Verification items for the finished model (mm, model axes). Round coordinates to 2 decimals unless told otherwise and drop trailing zeros. Order: outer loops, then holes, each group sorted by start corner. A loop starts at its lowest first (then second) coordinate and runs counter-clockwise, first axis right, second up. Notation, with made-up numbers: M 65.25,36.5 L 87.25,36.5 A18 cw 87.25,69.5 Z; hole C -28.5,-5.75 d7. An arc over 180 degrees is marked long. One line per item, written item: value. Start each with the question number.
from build123d import *

# Parameters (mm, degrees)
F1_DEPTH = 1.25
F2_R     = 2.5
F3_DEPTH = 2.501


# Not quite as in the source:
# - a feature names something its author has since deleted; it is built from what else it names


with BuildPart() as f1:
    # F0 (on Top) → F1 (new body, symmetric)
    with BuildSketch(Plane.XY):
        with BuildLine():
            Line((-5, 10), (-5, 0))
            Line((-5, 0), (5, 0))
            Line((5, 0), (5, 10))
            ThreePointArc((5, 10), (0, 5), (-5, 10))
        make_face()
        with BuildLine():
            Line((5, 0), (-5, 0))
            Line((-5, 0), (-5, -10))
            ThreePointArc((-5, -10), (0, -5), (5, -10))
            Line((5, -10), (5, 0))
        make_face()
        with BuildLine():
            ThreePointArc((5, 10), (0, 15), (-5, 10))
            ThreePointArc((-5, 10), (0, 5), (5, 10))
        make_face()
        with BuildLine():
            ThreePointArc((5, -10), (0, -5), (-5, -10))
            ThreePointArc((-5, -10), (0, -15), (5, -10))
        make_face()
    extrude(amount=F1_DEPTH, both=True)

    # F2 (on face) → F3 (cut, through all)
    with BuildSketch(Plane.XY.offset(1.25)):
        Circle(F2_R)
    extrude(amount=-F3_DEPTH, mode=Mode.SUBTRACT)


solid = f1.part
1. Depth check by flat-ended pin: pin 1 (4.5 mm diameter, centred on x = 0, y = 0, fed in from -Z). Enter the tip coordinate at first touch or a pass-through.
2. Draft check along Y on faces 1 (the face through (3, 0, -1.25)), 2 (the face through (-0.54, -2.44, 0.02)), 3 (the face through (0, 15, 0)), 4 (the face through (0, -15, 0)). Enter one of: released by +Y, released by -Y, zero draft, split by the parting line, or undercut.
3. Section check C-C (z = 0.7). Record the cut outline in (x, y), and give its area (3 significant figures).
4. Scan lines: line 1 along Y through (x, z) = (0, -0.5); line 2 along Y through (x, z) = (-2, 1); line 3 along X through (y, z) = (-0.5, -0.15). Record each from-to range of solid material in increasing order.
5. Section check B-B (y = 0). Record the cut outline in (x, z).
6. Section check D-D (x = -4.25). Record the cut outline in (y, z).
7. Section check A-A (x = 0). Record the cut outline in (y, z), and give its area (3 significant figures).
Geometry check:
1. pin 1: passes through
2. face 1: zero draft
2. face 2: undercut
2. face 3: released by +Y
2. face 4: released by -Y
3. outline: M -5,-10 A5 ccw 5,-10 L 5,10 A5 ccw -5,10 Z; hole C 0,0 d5
3. area: 259 mm²
4. line 1: y = -15 to -2.5, 2.5 to 15
4. line 2: y = -14.58 to -1.5, 1.5 to 14.58
4. line 3: x = -5 to -2.45, 2.45 to 5
5. outline: M -5,-1.25 L -2.5,-1.25 L -2.5,1.25 L -5,1.25 Z; M 2.5,-1.25 L 5,-1.25 L 5,1.25 L 2.5,1.25 Z
6. outline: M -12.63,-1.25 L 12.63,-1.25 L 12.63,1.25 L -12.63,1.25 Z
7. outline: M -15,-1.25 L -2.5,-1.25 L -2.5,1.25 L -15,1.25 Z; M 2.5,-1.25 L 15,-1.25 L 15,1.25 L 2.5,1.25 Z
7. area: 62.5 mm²
